Read the model definition and answer for the solid it produces. Units are mm, in the model's axes. A direction names the side the tool comes from. Round coordinates to 2 decimals unless told otherwise and drop trailing zeros. Order: outer loops, then holes, each group sorted by start corner. A loop starts at its lowest first (then second) coordinate and runs counter-clockwise, first axis right, second up. Notation, with made-up numbers: (89.5, 49) -> (108.5, 49) arc R29 ccw to (108.5, 73) -> close; hole circle Ø1 at (60, 45.5). An arc over 180 degrees is marked (long way). One line per item, written item: value. Start each with the question number.
1. For faces 1 (the face through (3.9, -0.9, -1.7)), 2 (the face through (12.5, -2, -0.5)), determine the directions among +Z, -Z, +X, -X, +Y, -Y from which every point of the face is accessible in a straight line to the end or side of a thin tool.
2. A flat-ended cylindrical pin translates along its axis: pin 1 Ø1.8 at (x, z) = (6, -2) entering from +Y. Find the tip coordinate at first contact, or state that the pin passes through.
3. Section C-C (z = -2.35) is taken. Give the vertices of the cut face in (x, y).
4. Section D-D (y = -3.3) is taken. Give the vertices of the cut face in (x, z), then the cut area to 3 significant figures.
5. The mould has two halves that part along X. Classify faces 3 (the face through (13, -2, -2)), 4 (the face through (0.5, -2, -3)), 5 (the face through (6, -1.9, -2)), 6 (the face through (6, -4, -2)): released by +X, released by -X, zero draft, split by the parting line, or undercut.
6. Section B-B (x = 7.25) is taken. Give the vertices of the cut face in (y, z).
7. Section A-A (y = -1.2) is taken. Give the vertices of the cut face in (x, z).
8. Consider line 1 (Y direction, x = 4.5, z = -2.8); line 2 (X direction, y = -0.65, z = -1.6); line 3 (X direction, y = -0.75, z = -2.95). Determine where each line is inside the solid, lowest interval first.
from build123d import *

# Parameters (mm, degrees)
F1_DEPTH = 4
F2_DEPTH = 1.9
F3_SIZE  = 1
F4_SIZE  = 0.2


with BuildPart() as f1:
    # F0 (on Front) → F1 (new body)
    with BuildSketch(Plane.XZ):
        with BuildLine():
            Line((4.5771115477, 0), (0, 0))
            Line((0, 0), (0, -3.5))
            Line((0, -3.5), (4.5771115477, -3.5))
            ThreePointArc((4.5771115477, -3.5), (3.9, -1.75), (4.5771115477, 0))
        make_face()
        with BuildLine():
            Line((8.4228884523, 0), (4.5771115477, 0))
            ThreePointArc((4.5771115477, 0), (3.9, -1.75), (4.5771115477, -3.5))
            Line((4.5771115477, -3.5), (8.4228884523, -3.5))
            ThreePointArc((8.4228884523, -3.5), (8.9248206094, -2.6882137347), (9.1, -1.75))
            ThreePointArc((9.1, -1.75), (8.9248206094, -0.8117862653), (8.4228884523, 0))
        make_face()
        with BuildLine():
            Line((13, 0), (8.4228884523, 0))
            ThreePointArc((8.4228884523, 0), (8.9248206094, -0.8117862653), (9.1, -1.75))
            ThreePointArc((9.1, -1.75), (8.9248206094, -2.6882137347), (8.4228884523, -3.5))
            Line((8.4228884523, -3.5), (13, -3.5))
            Line((13, -3.5), (13, 0))
        make_face()
    extrude(amount=F1_DEPTH)

    # F0 (on Front) → F2 (cut)
    with BuildSketch(Plane.XZ):
        with BuildLine():
            Line((8.4228884523, 0), (4.5771115477, 0))
            ThreePointArc((4.5771115477, 0), (3.9, -1.75), (4.5771115477, -3.5))
            Line((4.5771115477, -3.5), (8.4228884523, -3.5))
            ThreePointArc((8.4228884523, -3.5), (8.9248206094, -2.6882137347), (9.1, -1.75))
            ThreePointArc((9.1, -1.75), (8.9248206094, -0.8117862653), (8.4228884523, 0))
        make_face()
    extrude(amount=F2_DEPTH, mode=Mode.SUBTRACT)

    # F3
    f3_edges = [f1.edges().sort_by_distance(p)[0] for p in [
        (13, -2, -3.5),
        (13, -2, 0),
        (0, -2, -3.5),
        (0, -2, 0),
    ]]
    chamfer(f3_edges, length=F3_SIZE)

    # F4
    f4_edges = [f1.edges().sort_by_distance(p)[0] for p in [
        (6.5, -4, -3.5),
        (6.5, -4, 0),
    ]]
    chamfer(f4_edges, length=F4_SIZE)


solid = f1.part
Answer:
1. face 1: +Y
1. face 2: +Z, +X, +Y, -Y
2. pin 1: y = -1.9
3. outline: (0, -4) -> (13, -4) -> (13, 0) -> (9.03, 0) -> (9.03, -1.9) -> (3.97, -1.9) -> (3.97, 0) -> (0, 0) -> close
4. outline: (0, -2.5) -> (1, -3.5) -> (12, -3.5) -> (13, -2.5) -> (13, -1) -> (12, 0) -> (1, 0) -> (0, -1) -> close
4. area: 43.5 mm^2
5. face 3: released by +X
5. face 4: released by -X
5. face 5: undercut
5. face 6: zero draft
6. outline: (-4, -3.3) -> (-3.8, -3.5) -> (-1.9, -3.5) -> (-1.9, 0) -> (-3.8, 0) -> (-4, -0.2) -> close
7. outline: (0, -2.5) -> (1, -3.5) -> (4.58, -3.5) arc R2.6 cw to (4.58, 0) -> (1, 0) -> (0, -1) -> close; (8.42, -3.5) -> (12, -3.5) -> (13, -2.5) -> (13, -1) -> (12, 0) -> (8.42, 0) arc R2.6 cw to start
8. line 1: -4 to -1.9
8. line 2: 0 to 3.9, 9.1 to 13
8. line 3: 0.45 to 4.19, 8.81 to 12.55
